Can you work these out from the model? Positions are in its coordinate system, mm. A direction names the side the tool comes from. Round coordinates to 2 decimals unless told otherwise and drop trailing zeros. Order: outer loops, then holes, each group sorted by start corner. A loop starts at its lowest first (then second) coordinate and runs counter-clockwise, first axis right, second up. Notation, with made-up numbers: M 18,8 L 67,8 A10 ccw 67,23 Z; hole C -28.5,22.5 d6. An arc over 180 degrees is marked long. Answer as a JSON object with one key per item and string values. Group by question number.
Autodesk Inventor part; units mm, degrees
ref_plane "YZ Plane" through (0, 0, 0) normal (1, 0, 0) x (0, 1, 0)
ref_plane "XZ Plane" through (0, 0, 0) normal (0, 1, 0) x (-1, 0, 0)
ref_plane "XY Plane" through (0, 0, 0) normal (0, 0, 1) x (1, 0, 0)
sketch "Boceto1" plane through (0, 0, 0) normal (0, 1, 0) x (-1, 0, 0)
  line L0 (0, 12) -> (-3, 12)
  line L1 (-3, 12) -> (0, 12)
  line L2 (0, 12) -> (3, 12)
  line L3 (3, 12) -> (3, 9)
  line L4 (3, 9) -> (-3, 9)
  line L5 (-3, 9) -> (-3, 12)
  line L6 (0, -12) -> (-3, -12)
  line L7 (-3, -12) -> (-3, -9)
  line L8 (-3, -9) -> (3, -9)
  line L9 (3, -9) -> (3, -12)
  line L10 (3, -12) -> (-3, -12)
  point P0 (0, 0)
extrude "Extrusión1" add sketch "Boceto1" along normal blind 15
fillet "Empalme1" radius 3 4 edges at (3, 15, 10.5) (-3, 15, 10.5) (3, 15, -10.5) (-3, 15, -10.5)
sketch "Boceto2" plane through (0, 0, 0) normal (0, -1, 0) x (1, 0, 0)
  line L0 (-3, 9) -> (-3, 12)
  line L1 (3, -9) -> (3, -12)
  line L2 (-3, 12) -> (3, 12)
  line L3 (3, 12) -> (3, -12)
  line L4 (3, -12) -> (-3, -12)
  line L5 (-3, -12) -> (-3, 12)
  line L6 (3, 0) -> (3, -37.5)
  line L7 (3, 0) -> (3, 37.5)
  line L8 (3, 37.5) -> (-3, 37.5)
  line L9 (-3, 37.5) -> (-3, -37.5)
  line L10 (-3, -37.5) -> (3, -37.5)
  point P0 (0, 0)
  dimension "d11" = 37.5
  dimension "d12" = 37.5
extrude "Extrusión2" add sketch "Boceto2" along normal blind 3.5
sketch "Boceto3" plane through (0, -3.5, 0) normal (0, -1, 0) x (1, 0, 0)
  line L0 (-3, 37.5) -> (-3, -37.5)
  line L1 (3, -37.5) -> (3, 37.5)
  line L2 (-3, 37.5) -> (3, 37.5)
  line L3 (3, 37.5) -> (3, 40)
  line L4 (3, 40) -> (-3, 40)
  line L5 (-3, 40) -> (-3, 37.5)
  line L6 (-3, -37.5) -> (3, -37.5)
  line L7 (3, -37.5) -> (3, -40)
  line L8 (3, -40) -> (-3, -40)
  line L9 (-3, -40) -> (-3, -37.5)
  point P0 (0, 0)
  dimension "d15" = 2.5
  dimension "d16" = 2.5
extrude "Extrusión3" add sketch "Boceto3" along normal blind 12 contours L5 L4 L3 L2 | L6 L7 L8 L9
sketch "Boceto4" plane through (0, -3.5, 0) normal (0, 1, 0) x (1, 0, 0)
  line L0 (3, -40) -> (-3, -40)
  line L1 (3, 37.5) -> (3, -37.5)
  line L2 (-3, -40) -> (3, -40)
  line L3 (3, -40) -> (3, -37.5)
  line L4 (3, -37.5) -> (-3, -37.5)
  line L5 (-3, -37.5) -> (-3, -40)
  line L6 (-3, -37.5) -> (-3, 37.5)
  line L7 (-3, 40) -> (3, 40)
  line L8 (-3, 37.5) -> (3, 37.5)
  line L9 (3, 37.5) -> (3, 40)
  line L10 (3, 40) -> (-3, 40)
  line L11 (-3, 40) -> (-3, 37.5)
  point P0 (0, 0)
extrude "Extrusión4" add sketch "Boceto4" along normal blind 3.5 contours L0 L5 L4 L3 | L8 L11 L7 L9
sketch "Boceto5" plane through (-3, -15.5, 40) normal (0, 0, 1) x (1, 0, 0)
  line L0 (0, 0) -> (6, 0)
  line L1 (0, 15.5) -> (0, 0)
  line L2 (6, 0) -> (0, 0)
  line L3 (0, 0) -> (0, 3.5)
  line L4 (0, 3.5) -> (6, 3.5)
  line L5 (6, 3.5) -> (6, 0)
  point P0 (3, 15.5)
  dimension "d21" = 3.5
extrude "Extrusión5" add sketch "Boceto5" along normal blind 9
sketch "Boceto6" plane through (3, -15.5, -40) normal (0, 0, -1) x (-1, 0, 0)
  line L0 (6, 0) -> (0, 0)
  line L1 (0, 12) -> (0, 0)
  line L2 (6, 0) -> (0, 0)
  line L3 (0, 0) -> (0, 3.5)
  line L4 (0, 3.5) -> (6, 3.5)
  line L5 (6, 3.5) -> (6, 0)
  point P0 (3, 15.5)
  dimension "d24" = 3.5
extrude "Extrusión6" add sketch "Boceto6" along normal blind 9
sketch "Boceto7" plane through (0, 12, 12) normal (0, 0, 1) x (1, 0, 0)
  circle A0 centre (0, 0) radius 1.5
  point P0 (0, -12)
  dimension "d27" = 3
extrude "Extrusión7" cut sketch "Boceto7" against normal blind 31.25
sketch "Boceto8" plane through (-3, -12, 40) normal (0, 1, 0) x (1, 0, 0)
  line L0 (0, -9) -> (6, -9)
  line L1 (3, -9) -> (3, 0)
  line L2 (0, 0) -> (6, 0)
  line L3 (3, -4.5) -> (4.913, -4.5)
  line L4 (6, 80) -> (0, 80)
  line L5 (3, 80) -> (3, 89.023)
  line L6 (3, 84.5115) -> (4.913, 84.5115)
  point P0 (3, 40)
hole "Agujero1" at (0, -12, -44.5115) at (0, -12, 44.5) direction (0, -1, 0) diameter 2.9 depth 10 counterbore diameter 4 counterbore depth 2
properties part number "ventilador emergència inferior"
1) If we section it at D-D on y = -1: Write out the boundary of the cut face in (x, z), plus the area to 3 significant figures.
2) Which directions (+Z, -Z, +X, -X, +Y, -Y) give clear straight access to the entire face, cutting with the end or side of a thin tool? Please do faces 5 (the face through (0, -12, 42)), 6 (the face through (-1, -14, -43)), 7 (the face through (0, 0, 0)), 8 (the face through (0, -6, -40)), 9 (the face through (0, -3.5, 1)).
3) I need wall thicknesses on line 1 along Z through (x, y) = (0, -15.15); line 2 along Z through (x, y) = (0, -13.1); line 3 along Y through (x, z) = (0, -10.2). Which ranges of each line are inside material? Lowest first, please.
4) If we section it at A-A on z = 44.5: Write out the boundary of the cut face in (x, y), plus the area to 3 significant figures.
5) For pin 1 (1.8 mm diameter, centred on x = 0, y = -6, fed in from +Z); pin 2 (2.5 mm diameter, centred on x = 0, z = 44.5, fed in from -Y); pin 3 (3 mm diameter, centred on x = 2, z = 12, fed in from +Y); pin 4 (1.8 mm diameter, centred on x = -1, y = 10, fed in from -Z), each with a flat end and sliding along its axis, tell me the tip position at first contact or that it passes through.
6) We'd pull the mould along Z, two halves only. Please class faces 1 (the face through (0, 7, 9)), 2 (the face through (0, 7, 12)), 3 (the face through (-0.06, -14.76, -45.96)), 4 (the face through (-2.14, 14.1, -10.52)): +Z half, -Z half, draft (parallel to the pull), parting line (faces both ways), or undercut.
7) If we section it at B-B on y = 6: Write out the boundary of the cut face in (x, z), plus the area to 3 significant figures.
8) If we section it at C-C on z = 17.5: Write out the boundary of the cut face in (x, y).
Findings:
{
 "1": {"outline": "M -3,-40 L 3,-40 L 3,40 L -3,40 Z", "area": "480 mm^2"},
 "2": {"face 5": "+Z, +X, -X, +Y", "face 6": "+Y", "face 7": "+X, -X, +Y", "face 8": "-Z, +X, -X, +Y", "face 9": "+X, -X, -Y"},
 "3": {"line 1": "z = -49 to -45.96, -43.06 to -37.5, 37.5 to 43.05, 45.95 to 49", "line 2": "z = -49 to -46.51, -42.51 to -37.5, 37.5 to 42.5, 46.5 to 49", "line 3": "y = -3.5 to 10.5, 13.5 to 15"},
 "4": {"outline": "M -3,-15.5 L -1.45,-15.5 L -1.45,-14 L -2,-14 L -2,-12 L -3,-12 Z; M 1.45,-15.5 L 3,-15.5 L 3,-12 L 2,-12 L 2,-14 L 1.45,-14 Z", "area": "8.65 mm^2"},
 "5": {"pin 1": "stops at z = 40", "pin 2": "passes through", "pin 3": "stops at y = 14.96", "pin 4": "stops at z = -12"},
 "6": {"face 1": "undercut", "face 2": "+Z half", "face 3": "undercut", "face 4": "draft"},
 "7": {"outline": "M -3,-12 L 3,-12 L 3,-9 L -3,-9 Z; M -3,9 L 3,9 L 3,12 L -3,12 Z", "area": "36.0 mm^2"},
 "8": {"outline": "M -3,-3.5 L 3,-3.5 L 3,0 L -3,0 Z"}
}
